Autodesk Inventor part; units mm, degrees
ref_plane "YZ Plane" through (0, 0, 0) normal (1, 0, 0) x (0, 1, 0)
ref_plane "XZ Plane" through (0, 0, 0) normal (0, 1, 0) x (-1, 0, 0)
ref_plane "XY Plane" through (0, 0, 0) normal (0, 0, 1) x (1, 0, 0)
ref_plane "Arbeitsebene1" through (0, 0, 0) normal (0, 0, 1) x (1, 0, 0)
sketch "Skizze1" plane through (0, 0, 0) normal (0, 0, 1) x (1, 0, 0)
  arc A0 (13.4381, 5.6873) -> (13.3881, 5.2) centre (15.7881, 5.2) ccw construction
  line L0 (13.4381, 5.6873) -> (13.4381, 7.6) construction
  line L1 (13.4381, 7.6) -> (15.7881, 7.6) construction
  arc A1 (18.1881, 5.2) -> (15.7881, 7.6) centre (15.7881, 5.2) ccw
  line L2 (18.1881, 5.2) -> (18.1881, -5.2) construction
  arc A2 (15.7881, -7.6) -> (18.1881, -5.2) centre (15.7881, -5.2) ccw
  line L3 (15.7881, -7.6) -> (13.4381, -7.6) construction
  line L4 (13.4381, -7.6) -> (13.4381, -5.6873) construction
  arc A3 (13.3881, -5.2) -> (13.4381, -5.6873) centre (15.7881, -5.2) ccw construction
  line L5 (13.3881, -5.2) -> (13.3881, 5.2) construction
  arc A4 (14.5, 9) -> (11.5, 6) centre (14.5, 6) ccw construction
  line L6 (11.5, -6) -> (11.5, 6) construction
  arc A5 (11.5, -6) -> (14.5, -9) centre (14.5, -6) ccw construction
  line L7 (14.9, -9) -> (14.5, -9) construction
  arc A6 (17.9, -12) -> (14.9, -9) centre (14.9, -12) ccw
  line L8 (17.9, -12) -> (17.9, -21.066)
  line L9 (6.7383, -21.066) -> (-6.9383, -21.066)
  line L10 (-17.9, -21.066) -> (-17.9, 21.066)
  line L11 (-17.9, 21.066) -> (17.9, 21.066)
  line L12 (17.9, 21.066) -> (17.9, 12)
  arc A7 (14.9, 9) -> (17.9, 12) centre (14.9, 12) ccw
  line L13 (14.5, 9) -> (14.9, 9) construction
  circle A8 centre (-20, 20) radius 1.6 construction
  circle A9 centre (20, -20) radius 1.6 construction
  circle A10 centre (-20, -20) radius 1.6 construction
  circle A11 centre (20, 20) radius 1.6 construction
  arc A12 (-22.9, 24.9) -> (-24.9, 22.9) centre (-22.9, 22.9) ccw
  line L14 (-24.9, 22.9) -> (-24.9, -22.9)
  arc A13 (-24.9, -22.9) -> (-22.9, -24.9) centre (-22.9, -22.9) ccw
  line L15 (-22.9, -24.9) -> (22.9, -24.9)
  arc A14 (22.9, -24.9) -> (24.9, -22.9) centre (22.9, -22.9) ccw
  line L16 (24.9, -22.9) -> (24.9, 22.9)
  arc A15 (24.9, 22.9) -> (22.9, 24.9) centre (22.9, 22.9) ccw
  line L17 (22.9, 24.9) -> (-22.9, 24.9)
  arc A16 (6.7383, -21.066) -> (8.3017, -21.066) centre (7.52, -20.62) ccw
  arc A17 (-8.5017, -21.066) -> (-6.9383, -21.066) centre (-7.72, -20.62) ccw
  line L18 (-8.5017, -21.066) -> (-17.9, -21.066)
  line L19 (17.9, -21.066) -> (8.3017, -21.066)
  line L20 (17.9, -12) -> (17.9, 12)
  circle A18 centre (-20, 20) radius 1.4
  line L21 (-20, 20) -> (20, 20) construction
  line L22 (20, 20) -> (20, -20) construction
  line L23 (20, -20) -> (-20, -20) construction
  line L24 (-20, -20) -> (-20, 20) construction
  circle A19 centre (20, -20) radius 1.4
  circle A20 centre (20, 20) radius 1.4
  circle A21 centre (-20, -20) radius 1.4
  line L25 (25.9, -32.5) -> (25.9, 32.5)
  line L26 (22.9, -24.9) -> (25.9, -24.9)
  line L27 (22.9, 24.9) -> (25.9, 24.9)
  point P0 (0, 0)
  dimension "d7" = 2.8
  dimension "d8" = 40
  dimension "d9" = 40
  dimension "d10" = 2.8
  dimension "d11" = 2.8
  dimension "d12" = 2.8
extrude "Extrusion1" add sketch "Skizze1" along normal blind 5
sketch "Sketch6" plane through (25.9, -24.9, 0) normal (1, 0, 0) x (0, 0, -1)
  circle A0 centre (-16.9, 25) radius 22.5
  circle A1 centre (-16.9, 25) radius 15.75
  line L0 (-5, 0) -> (-5, 49.8)
  line L1 (-5, 14.6824) -> (-5, 5.9045)
  line L2 (-5, 44.0955) -> (-5, 35.3176)
  arc A2 (-5, 46.8294) -> (-5, 3.1706) centre (-16.9, 25) ccw
  line L3 (-5, 46.8294) -> (-5, 35.3176)
  line L4 (-5, 14.6824) -> (-5, 3.1706)
  point P0 (0, 24.9)
extrude "Extrusion3" add sketch "Sketch6" against normal blind 4 contours L0 A1 A0 | A0 L0 A2 picked at (-36.9413, 23.2431)
sketch "Sketch7" plane through (21.9, -24.9, 0) normal (-1, 0, 0) x (0, 0, 1)
  circle A0 centre (2.9774, 8.4941) radius 0.25
  circle A1 centre (16.8445, 3.4065) radius 0.25
  circle A2 centre (30.7375, 8.4227) radius 0.25
  circle A3 centre (38.1558, 21.1956) radius 0.25
  circle A4 centre (35.6283, 35.7487) radius 0.25
  circle A5 centre (24.3376, 45.2723) radius 0.25
  circle A6 centre (9.5668, 45.3103) radius 0.25
  circle A7 centre (-1.7728, 35.8449) radius 0.25
  circle A8 centre (-4.3751, 21.305) radius 0.25
  line L0 (-2.665, 15.2234) -> (2.0334, 16.9335)
  line L1 (2.0334, 16.9335) -> (0.3233, 21.632)
  line L2 (0.3233, 21.632) -> (-4.3751, 19.9219)
  line L3 (-4.3751, 19.9219) -> (-2.665, 15.2234)
  line L4 (1.8587, 9.1214) -> (5.6889, 12.3353)
  line L5 (5.6889, 12.3353) -> (2.4749, 16.1656)
  line L6 (2.4749, 16.1656) -> (-1.3553, 12.9516)
  line L7 (-1.3553, 12.9516) -> (1.8587, 9.1214)
  line L8 (8.1966, 4.9346) -> (10.6966, 9.2647)
  line L9 (10.6966, 9.2647) -> (6.3664, 11.7647)
  line L10 (6.3664, 11.7647) -> (3.8664, 7.4346)
  line L11 (3.8664, 7.4346) -> (8.1966, 4.9346)
  line L12 (15.5842, 3.1679) -> (16.4525, 8.0919)
  line L13 (16.4525, 8.0919) -> (11.5284, 8.9602)
  line L14 (11.5284, 8.9602) -> (10.6602, 4.0361)
  line L15 (10.6602, 4.0361) -> (15.5842, 3.1679)
  line L16 (23.1306, 4.0345) -> (22.2623, 8.9586)
  line L17 (22.2623, 8.9586) -> (17.3383, 8.0903)
  line L18 (17.3383, 8.0903) -> (18.2066, 3.1663)
  line L19 (18.2066, 3.1663) -> (23.1306, 4.0345)
  line L20 (29.9255, 7.4299) -> (27.4255, 11.76)
  line L21 (27.4255, 11.76) -> (23.0953, 9.26)
  line L22 (23.0953, 9.26) -> (25.5953, 4.9299)
  line L23 (25.5953, 4.9299) -> (29.9255, 7.4299)
  line L24 (35.1493, 12.9445) -> (31.319, 16.1584)
  line L25 (31.319, 16.1584) -> (28.1051, 12.3282)
  line L26 (28.1051, 12.3282) -> (31.9353, 9.1142)
  line L27 (31.9353, 9.1142) -> (35.1493, 12.9445)
  line L28 (38.1719, 19.9131) -> (33.4735, 21.6232)
  line L29 (33.4735, 21.6232) -> (31.7634, 16.9247)
  line L30 (31.7634, 16.9247) -> (36.4618, 15.2146)
  line L31 (36.4618, 15.2146) -> (38.1719, 19.9131)
  line L32 (38.6289, 27.4953) -> (33.6289, 27.4953)
  line L33 (33.6289, 27.4953) -> (33.6289, 22.4953)
  line L34 (33.6289, 22.4953) -> (38.6289, 22.4953)
  line L35 (38.6289, 22.4953) -> (38.6289, 27.4953)
  line L36 (36.465, 34.7766) -> (31.7666, 33.0665)
  line L37 (31.7666, 33.0665) -> (33.4767, 28.368)
  line L38 (33.4767, 28.368) -> (38.1751, 30.0781)
  line L39 (38.1751, 30.0781) -> (36.465, 34.7766)
  line L40 (31.9413, 40.8786) -> (28.1111, 37.6647)
  line L41 (28.1111, 37.6647) -> (31.3251, 33.8344)
  line L42 (31.3251, 33.8344) -> (35.1553, 37.0484)
  line L43 (35.1553, 37.0484) -> (31.9413, 40.8786)
  line L44 (25.6034, 45.0654) -> (23.1034, 40.7353)
  line L45 (23.1034, 40.7353) -> (27.4336, 38.2353)
  line L46 (27.4336, 38.2353) -> (29.9336, 42.5654)
  line L47 (29.9336, 42.5654) -> (25.6034, 45.0654)
  line L48 (18.2158, 46.8321) -> (17.3475, 41.9081)
  line L49 (17.3475, 41.9081) -> (22.2716, 41.0398)
  line L50 (22.2716, 41.0398) -> (23.1398, 45.9639)
  line L51 (23.1398, 45.9639) -> (18.2158, 46.8321)
  line L52 (10.6694, 45.9655) -> (11.5377, 41.0414)
  line L53 (11.5377, 41.0414) -> (16.4617, 41.9097)
  line L54 (16.4617, 41.9097) -> (15.5934, 46.8337)
  line L55 (15.5934, 46.8337) -> (10.6694, 45.9655)
  line L56 (3.8745, 42.5701) -> (6.3745, 38.24)
  line L57 (6.3745, 38.24) -> (10.7047, 40.74)
  line L58 (10.7047, 40.74) -> (8.2047, 45.0701)
  line L59 (8.2047, 45.0701) -> (3.8745, 42.5701)
  line L60 (-1.3493, 37.0555) -> (2.481, 33.8416)
  line L61 (2.481, 33.8416) -> (5.6949, 37.6718)
  line L62 (5.6949, 37.6718) -> (1.8647, 40.8858)
  line L63 (1.8647, 40.8858) -> (-1.3493, 37.0555)
  line L64 (-4.3719, 30.0869) -> (0.3265, 28.3768)
  line L65 (0.3265, 28.3768) -> (2.0366, 33.0753)
  line L66 (2.0366, 33.0753) -> (-2.6618, 34.7854)
  line L67 (-2.6618, 34.7854) -> (-4.3719, 30.0869)
  line L68 (-4.8289, 22.5047) -> (0.1711, 22.5047)
  line L69 (0.1711, 22.5047) -> (0.1711, 27.5047)
  line L70 (0.1711, 27.5047) -> (-4.8289, 27.5047)
  line L71 (-4.8289, 27.5047) -> (-4.8289, 22.5047)
  circle A9 centre (16.9, 25) radius 15.75
  circle A10 centre (16.9, 25) radius 22.5
  point P0 (0, 24.9)
hole "Hole1" at (21.9, 20.4103, 9.5668) at (21.9, 20.3723, 24.3376) at (21.9, 10.8487, 35.6283) at (21.9, -3.7044, 38.1558) at (21.9, -16.4773, 30.7375) at (21.9, -21.4935, 16.8445) direction (1, 0, 0) diameter 2 end through all
fillet "Fillet2" radius 3.2 2 edges at (21.9, 16.1735, 5) (21.9, -15.9735, 5)
properties part number "30_Cube_LED_Array_v0"
Geometry check sheet. Reference: the model listing, model coordinates, mm. A direction names the side the tool comes from. Round coordinates to 2 decimals unless told otherwise and drop trailing zeros. Loops run counter-clockwise (first coordinate to the right, second up) from the corner with the lowest first, then second, coordinate; pieces in that order, holes last. Notation, with made-up numbers: (47.5, 8) -> (91.5, 8) arc R28 cw to (91.5, 45) -> close; hole circle Ø10 at (21, 36). An arc over 180 degrees is marked (long way). Answer as a JSON object with one key per item and string values. Group by question number.
Item 1: Cross-section at D-D, the plane x = -20. Record the cut outline in (y, z).
Item 2: Thickness scan on line 1 along Y through (x, z) = (20, 4); line 2 along X through (y, z) = (1, 2); line 3 along Y through (x, z) = (12, 2). Record the ranges inside material, lowest first.
Item 3: Cross-section at B-B, the plane y = 17.5. Record the cut outline in (x, z), plus the area to 3 significant figures.
Item 4: Set-up check for faces 1 (the face through (17.9, 0, 2)), 2 (the face through (23.93, 21.35, 24.12)), 3 (the face through (-18.4, 0.1, 5)): record each of +Z, -Z, +X, -X, +Y, -Y from which the full face is reachable in a straight line by a thin tool's end or side.
Item 5: Release check for a two-part mould opening along Y. For faces 4 (the face through (1, -24.9, 2)), 5 (the face through (-13, -21.066, 2)), 6 (the face through (-24.9, 0, 2)) record: pulls with the +Y half, pulls with the -Y half, needs draft (parallel to the pull), parting line crosses it, or undercut.
Item 6: Depth check by flat-ended pin: pin 1 Ø3 at (y, z) = (-3.7, 38.16) entering from -X; pin 2 Ø15 at (x, y) = (12, -7) entering from +Z; pin 3 Ø3 at (y, z) = (-13.5, 8) entering from -X. Enter the tip coordinate at first touch or a pass-through.
Item 7: Cross-section at C-C, the plane z = 14. Record the cut outline in (x, y), plus the area to 3 significant figures.
Item 8: Cross-section at A-A, the plane x = -2.5. Record the cut outline in (y, z), plus the area to 3 significant figures.
Determined:
{
 "1": {"outline": "(-24.9, 0) -> (-21.4, 0) -> (-21.4, 5) -> (-24.9, 5) -> close; (-18.6, 0) -> (18.6, 0) -> (18.6, 5) -> (-18.6, 5) -> close; (21.4, 0) -> (24.9, 0) -> (24.9, 5) -> (21.4, 5) -> close"},
 "2": {"line 1": "y = -24.9 to -21.4, -18.6 to 18.6, 21.4 to 24.9", "line 2": "x = -24.9 to -17.9, 17.9 to 25.9", "line 3": "y = -24.9 to -21.07, 21.07 to 24.9"},
 "3": {"outline": "(-24.9, 0) -> (-17.9, 0) -> (-17.9, 5) -> (-24.9, 5) -> close; (17.9, 0) -> (25.9, 0) -> (25.9, 34.66) -> (21.9, 34.66) -> (21.9, 8.2) arc R3.2 cw to (18.7, 5) -> (17.9, 5) -> close", "area": "196 mm²"},
 "4": {"face 1": "+Z, -Z", "face 2": "+X, -X", "face 3": "-X"},
 "5": {"face 4": "pulls with the -Y half", "face 5": "undercut", "face 6": "needs draft"},
 "6": {"pin 1": "stops at x = 21.9", "pin 2": "stops at z = 5", "pin 3": "stops at x = 21.41"},
 "7": {"outline": "(21.9, -24.59) -> (25.9, -24.59) -> (25.9, -15.38) -> (21.9, -15.38) -> close; (21.9, 15.58) -> (25.9, 15.58) -> (25.9, 24.79) -> (21.9, 24.79) -> close", "area": "73.7 mm²"},
 "8": {"outline": "(-24.9, 0) -> (-21.07, 0) -> (-21.07, 5) -> (-24.9, 5) -> close; (21.07, 0) -> (24.9, 0) -> (24.9, 5) -> (21.07, 5) -> close", "area": "38.3 mm²"}
}
